Could you check a few things on this model? Use its own coordinates, in mm. A direction names the side the tool comes from. Round coordinates to 2 decimals unless told otherwise and drop trailing zeros. Loops run counter-clockwise (first coordinate to the right, second up) from the corner with the lowest first, then second, coordinate; pieces in that order, holes last.
from build123d import *

# Parameters (mm, degrees)
SKETCH1_R           = 17.5
SKETCH1_R_2         = 6
BOSS_EXTRUDE1_DEPTH = 12
CUT_EXTRUDE1_START  = -6
SKETCH2_W           = 130
SKETCH2_H           = 70
CUT_EXTRUDE1_DEPTH  = 6


with BuildPart() as part:
    # Sketch1 → Boss-Extrude1 (new body)
    with BuildSketch(Plane(origin=(0, 0, 0), x_dir=(1, 0, 0), z_dir=(0, 1, 0))):
        Polygon((0, 0), (25, 0), (25, -60), (225, -60), (225, 0), (250, 0), (250, 25), (310, 25), (310, 125), (250, 125), (250, 150), (225, 150), (225, 210), (25, 210), (25, 150), (0, 150), (0, 125), (-60, 125), (-60, 25), (0, 25), align=None)
        with Locations(Location((75, 75, 0), (0, 0, 270))):
            Circle(SKETCH1_R, mode=Mode.SUBTRACT)
        with Locations(Location((33.5, 33.5, 0), (0, 0, 270))):
            Circle(SKETCH1_R_2, mode=Mode.SUBTRACT)
        with Locations(Location((116.5, 33.5, 0), (0, 0, 270))):
            Circle(SKETCH1_R_2, mode=Mode.SUBTRACT)
        with Locations(Location((116.5, 116.5, 0), (0, 0, 270))):
            Circle(SKETCH1_R_2, mode=Mode.SUBTRACT)
        with Locations(Location((33.5, 116.5, 0), (0, 0, 270))):
            Circle(SKETCH1_R_2, mode=Mode.SUBTRACT)
        with BuildLine():
            Line((-25.5, 100), (-25.5, 50))
            ThreePointArc((-25.5, 50), (-30, 45.5), (-34.5, 50))
            Line((-34.5, 50), (-34.5, 100))
            ThreePointArc((-34.5, 100), (-30, 104.5), (-25.5, 100))
        make_face(mode=Mode.SUBTRACT)
        with BuildLine():
            Line((50, 184.5), (200, 184.5))
            ThreePointArc((200, 184.5), (204.5, 180), (200, 175.5))
            Line((200, 175.5), (50, 175.5))
            ThreePointArc((50, 175.5), (45.5, 180), (50, 184.5))
        make_face(mode=Mode.SUBTRACT)
        with BuildLine():
            Line((50, -25.5), (200, -25.5))
            ThreePointArc((200, -25.5), (204.5, -30), (200, -34.5))
            Line((200, -34.5), (50, -34.5))
            ThreePointArc((50, -34.5), (45.5, -30), (50, -25.5))
        make_face(mode=Mode.SUBTRACT)
        with BuildLine():
            Line((275.5, 50), (275.5, 100))
            ThreePointArc((275.5, 100), (280, 104.5), (284.5, 100))
            Line((284.5, 100), (284.5, 50))
            ThreePointArc((284.5, 50), (280, 45.5), (275.5, 50))
        make_face(mode=Mode.SUBTRACT)
        with BuildLine():
            Line((147.5, 54.43), (242.5, 54.43))
            ThreePointArc((242.5, 54.43), (245.5, 51.43), (242.5, 48.43))
            Line((242.5, 48.43), (147.5, 48.43))
            ThreePointArc((147.5, 48.43), (144.5, 51.43), (147.5, 54.43))
        make_face(mode=Mode.SUBTRACT)
        with BuildLine():
            Line((147.5, 101.57), (242.5, 101.57))
            ThreePointArc((242.5, 101.57), (245.5, 98.57), (242.5, 95.57))
            Line((242.5, 95.57), (147.5, 95.57))
            ThreePointArc((147.5, 95.57), (144.5, 98.57), (147.5, 101.57))
        make_face(mode=Mode.SUBTRACT)
        with BuildLine():
            Line((147.5, 80), (242.5, 80))
            ThreePointArc((242.5, 80), (247.5, 75), (242.5, 70))
            Line((242.5, 70), (147.5, 70))
            ThreePointArc((147.5, 70), (142.5, 75), (147.5, 80))
        make_face(mode=Mode.SUBTRACT)
    extrude(amount=BOSS_EXTRUDE1_DEPTH)

    # Sketch2 → Cut-Extrude1 (cut)
    with BuildSketch(Plane(origin=(0, 0, 0), x_dir=(-1, 0, 0), z_dir=(0, -1, 0)).offset(CUT_EXTRUDE1_START)):
        with Locations((-195, 75)):
            Rectangle(SKETCH2_W, SKETCH2_H)
    extrude(amount=-CUT_EXTRUDE1_DEPTH, mode=Mode.SUBTRACT)


solid = part.part
Item 1: If I drill on line 1 along X through (y, z) = (4.75, -116.5); line 2 along X through (y, z) = (8.75, -117.5); line 3 along X through (y, z) = (9.25, -75), over which ranges is the centre line in solid material (lowest first)?
Results list:
line 1: x = -60 to 27.5, 39.5 to 110.5, 122.5 to 310
line 2: x = -60 to 27.58, 39.42 to 110.58, 122.42 to 310
line 3: x = -60 to -34.5, -25.5 to 57.5, 92.5 to 130, 260 to 275.5, 284.5 to 310
Item 2: If we section it at C-C, the plane x = 186: Please give me the cut outline in (y, z).
Results list:
outline: (0, -210) - (12, -210) - (12, -184.5) - (0, -184.5) - close; (0, -175.5) - (12, -175.5) - (12, -110) - (6, -110) - (6, -101.57) - (0, -101.57) - close; (0, -95.57) - (6, -95.57) - (6, -80) - (0, -80) - close; (0, -70) - (6, -70) - (6, -54.43) - (0, -54.43) - close; (0, -48.43) - (6, -48.43) - (6, -40) - (12, -40) - (12, 25.5) - (0, 25.5) - close; (0, 34.5) - (12, 34.5) - (12, 60) - (0, 60) - close
Item 3: If we section it at B-B, the plane z = 30: Please give me the cut outline in (x, y), then the cut area to 3 significant figures.
Results list:
outline: (25, 0) - (45.5, 0) - (45.5, 12) - (25, 12) - close; (204.5, 0) - (225, 0) - (225, 12) - (204.5, 12) - close
area: 492 mm2
Item 4: If we section it at A-A, the plane x = -30: Please give me the cut outline in (y, z), then the cut area to 3 significant figures.
Results list:
outline: (0, -125) - (12, -125) - (12, -104.5) - (0, -104.5) - close; (0, -45.5) - (12, -45.5) - (12, -25) - (0, -25) - close
area: 492 mm2
Item 5: For faces 1 (the flat face through (280, 6, -125)), 2 (the flat face through (250, 6, -12)), 3 (the flat face through (12, 6, 0)), 4 (the flat face through (275.5, 6, -75)), 5 (the flat face through (-30, 6, -125)), which set-ups out of +Z, -Z, +X, -X, +Y, -Y let a thin tool reach every point of the face, with its end or its side?
Results list:
face 1: -Z, +X, +Y, -Y
face 2: +Z, +X, +Y, -Y
face 3: +Z, -X, +Y, -Y
face 4: +Y, -Y
face 5: -Z, -X, +Y, -Y
Item 6: Will these pins go through, and if not, where does the flat tip stop? pin 1 (6 mm diameter, centred on y = 7.5, z = 31.5, fed in from +X); pin 2 (6 mm diameter, centred on y = 8, z = -142, fed in from -X).
Results list:
pin 1: stops at x = 225
pin 2: stops at x = 0
Item 7: If we section it at D-D, the plane z = -85: Please give me the cut outline in (x, y).
Results list:
outline: (-60, 0) - (-34.5, 0) - (-34.5, 12) - (-60, 12) - close; (-25.5, 0) - (60.64, 0) - (60.64, 12) - (-25.5, 12) - close; (89.36, 0) - (275.5, 0) - (275.5, 12) - (260, 12) - (260, 6) - (130, 6) - (130, 12) - (89.36, 12) - close; (284.5, 0) - (310, 0) - (310, 12) - (284.5, 12) - close
Item 8: We'd pull the mould along X, two halves only. Please class faces 6 (the flat face through (124, 6, -184.5)), 7 (the flat face through (250, 6, -137)), 8 (the cylindrical face through (59.474, 5.916, -66.925)), 9 (the flat face through (124, 6, 60)): released by +X, released by -X, zero draft, split by the parting line, or undercut.
Results list:
face 6: undercut
face 7: released by +X
face 8: undercut
face 9: zero draft
